Source: three-view drawing plus pictorial views. Frame: mm from the lowest corner of the part. A direction names the side the tool comes from. Give positions to 0.01 mm unless a question says otherwise; leave off trailing zeros. Order: outer loops, then holes, each group sorted by start corner. A loop starts at its lowest first (then second) coordinate and runs counter-clockwise, first axis right, second up. Notation, with made-up numbers: (9, 0.25) -> (36, 0.25) arc R19 ccw to (36, 36.25) -> close; hole circle Ø2 at (-3, 51). An arc over 180 degrees is marked (long way). One line per question, with ' | ' between items.
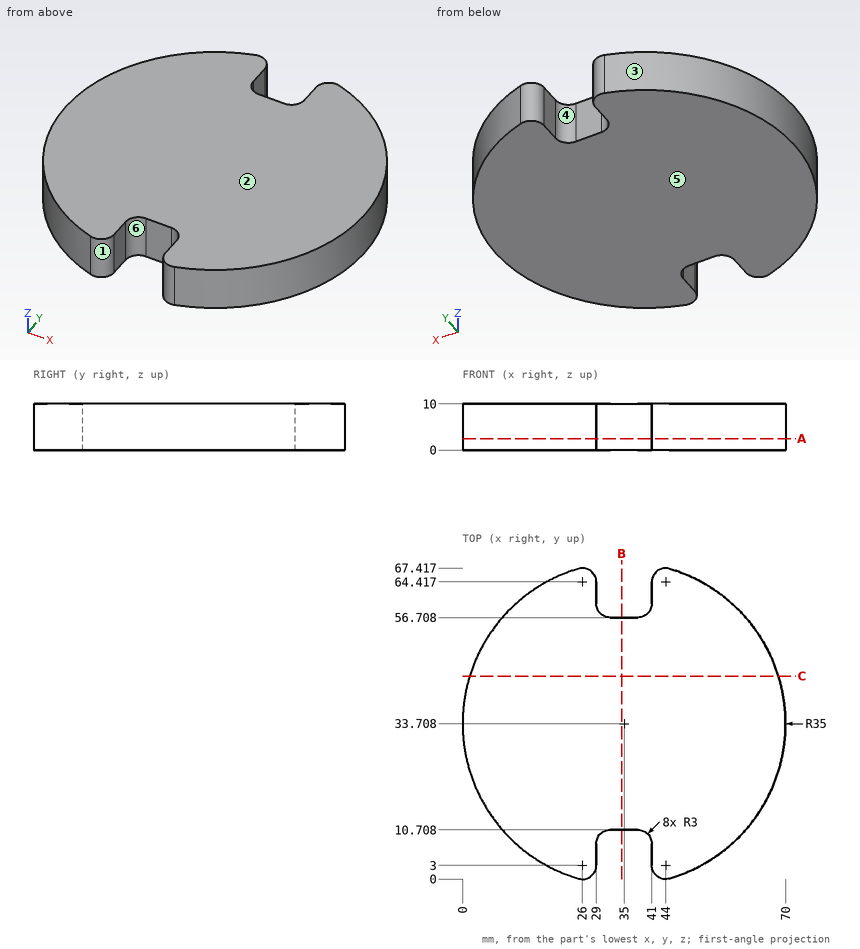
1) Contact query for flat-ended pins moving along their axis: pin 1 Ø4 at (y, z) = (61.5, 4.5) entering from +X; pin 2 Ø1.4 at (y, z) = (61.5, 6) entering from -X; pin 3 Ø5 at (y, z) = (4.5, 3) entering from -X; pin 4 Ø8 at (x, y) = (37, 18.5) entering from -Z. Output: stop coordinate, or through.
Check result:
pin 1: stops at x = 58.66 | pin 2: stops at x = 12.84 | pin 3: stops at x = 12.38 | pin 4: stops at z = 0
2) Section A-A on z = 2.5. Return loops of the section in (x, y) (1 decimal), plus the area to 3 significant figures.
Check result:
outline: (25.2, 0.1) arc R3 ccw to (29, 3) -> (29, 7.7) arc R3 cw to (32, 10.7) -> (38, 10.7) arc R3 cw to (41, 7.7) -> (41, 3) arc R3 ccw to (44.8, 0.1) arc R35 ccw to (44.8, 67.3) arc R3 ccw to (41, 64.4) -> (41, 59.7) arc R3 cw to (38, 56.7) -> (32, 56.7) arc R3 cw to (29, 59.7) -> (29, 64.4) arc R3 ccw to (25.2, 67.3) arc R35 ccw to start | area: 3,560 mm^2
3) Section B-B on x = 34.5. Return loops of the section in (y, z), plus the area to 3 significant figures.
Check result:
outline: (10.71, 0) -> (56.71, 0) -> (56.71, 10) -> (10.71, 10) -> close | area: 460 mm^2
4) Section C-C on y = 44. Return loops of the section in (x, z), plus the area to 3 significant figures.
Check result:
outline: (1.55, 0) -> (68.45, 0) -> (68.45, 10) -> (1.55, 10) -> close | area: 669 mm^2
5) Set-up query: the marked faces 4, 5 and 6. Return all of +Z, -Z, +X, -X, +Y, -Y with unobstructed straight access to the full face (end or side cutting, diameter ignored); none if empty.
Check result:
face 4: +Z, -Z, +Y | face 5: -Z, +X, -X, +Y, -Y | face 6: +Z, -Z, -Y
6) Pull-direction query (X, two-part tool) for the marked faces 1, 2 and 3; classes: +X half, -X half, draft (parallel to the pull), parting line (faces both ways), or undercut.
Check result:
face 1: undercut | face 2: draft | face 3: -X half
7) Material intervals for probe 1 along Y at (x, z) = (32, 9); probe 2 along X at (y, z) = (57.5, 7.5); probe 3 along X at (y, z) = (10, 7.75) (1 decimal), sorted ascending. Write a range as from..to.
Check result:
probe 1: y = 10.71..56.71 | probe 2: x = 9.33..29.97, 40.03..60.67 | probe 3: x = 9.3..30.1, 39.9..60.7
